```python
from build123d import *

# Parameters (mm, degrees)
BOSS_EXTRUDE1_DEPTH      = 47.625
BOSS_EXTRUDE1_DEPTH_BACK = 9.525
SKETCH2_R                = 9.525
CUT_EXTRUDE1_DEPTH       = 122.738617419


with BuildPart() as part:
    # Sketch1 → Boss-Extrude1 (new, two sides: drawn at the far end of the back side and taken through both)
    with BuildSketch(Plane.XY.offset(-BOSS_EXTRUDE1_DEPTH_BACK)):
        Polygon((-104.425717212, 293.558329543), (-143.022728413, 260.774121234), (-145.397980675, 262.922347723), (-106.481154517, 295.978206086), align=None)
    extrude(amount=BOSS_EXTRUDE1_DEPTH + BOSS_EXTRUDE1_DEPTH_BACK)

    # Sketch2 → Cut-Extrude1 (cut, through all)
    with BuildSketch(Plane(origin=(-188.610450601, 222.052019857, 0), x_dir=(0.762165840447724, 0.6473818283321017, 0), z_dir=(0.6473818283321017, -0.762165840447724, 0))):
        with Locations((85.054613578, 19.05)):
            Circle(SKETCH2_R)
        Polygon((110.454613578, -9.525), (88.229613578, -9.525), (88.229613578, -6.349999999), (91.404613578, -6.349999999), (91.404613578, -3.175), (97.754613578, -3.175), (97.754613578, 0), (110.454613578, 0), (113.679871945, 0), (113.679871945, -9.525), align=None)
        Polygon((59.813389382, -9.525), (82.038389382, -9.525), (82.038389382, -6.349999999), (78.863389382, -6.349999999), (78.863389382, -3.175), (72.513389382, -3.175), (72.513389382, 0), (59.813389382, 0), (54.830807426, 0), (54.830807426, -9.525), align=None)
        Polygon((110.454613578, 38.1), (118.192353476, 38.1), (118.192353476, 47.625), (110.454613578, 47.625), (88.229613578, 47.625), (88.229613578, 44.449999999), (91.404613578, 44.449999999), (91.404613578, 41.275), (97.754613578, 41.275), (97.754613578, 38.1), align=None)
        Polygon((59.393776038, 38.1), (50.339137781, 38.1), (50.339137781, 47.625), (59.393776038, 47.625), (81.618776038, 47.625), (81.618776038, 44.449999999), (78.443776038, 44.449999999), (78.443776038, 41.275), (72.093776038, 41.275), (72.093776038, 38.1), align=None)
    extrude(amount=-CUT_EXTRUDE1_DEPTH, mode=Mode.SUBTRACT)


solid = part.part
```
The listing builds one solid part. Answer for the finished solid, in the listing's coordinates (mm). A direction names the side the tool comes from. Round coordinates to 2 decimals unless told otherwise and drop trailing zeros. Loops run counter-clockwise (first coordinate to the right, second up) from the corner with the lowest first, then second, coordinate; pieces in that order, holes last.
1) For faces 1 (the face through (-127.1, 276.36, -7.96)), 2 (the face through (-118, 284, 41.275)), 3 (the face through (-118, 284, -3.175)), determine the directions among +Z, -Z, +X, -X, +Y, -Y from which every point of the face is accessible in a straight line to the end or side of a thin tool.
Outcome:
face 1: -Z, -X, -Y
face 2: +Z, +X, +Y
face 3: -Z, +X, +Y
2) Given P1, Ø7, axis at x = -116.5, y = 284.5, coming from the +Z side (3 decimals); P2, Ø7, axis at x = -119, y = 285, coming from the -Z side; P3, Ø8.5, axis at x = -108.5, y = 290.5, coming from the -Z side, each flat-ended and moving along its own axis, determine where each tip first touches the part or whether it passes through.
Outcome:
P1: stops at z = 41.275
P2: stops at z = -6.35
P3: stops at z = 0
3) A cutting plane is placed at D-D on y = 264.5. Determine the outline of the cut face in (x, z), plus the area to 3 significant figures.
Outcome:
outline: (-143.54, 0) - (-138.64, 0) - (-138.64, 38.1) - (-143.54, 38.1) - close
area: 187 mm2
4) Consider line 1 (Z direction, x = -133, y = 273) (3 decimals); line 2 (Y direction, x = -134, z = 33); line 3 (X direction, y = 286.5, z = 25). Determine where each line is inside the solid, lowest interval first.
Outcome:
line 1: z = -3.175 to 41.275
line 2: y = 268.44 to 272.6
line 3: x = -117.64 to -112.74
5) A cutting plane is placed at B-B on x = -115.5. Determine the outline of the cut face in (y, z) (3 decimals).
Outcome:
outline: (284.152, -3.175) - (286.979, -3.175) - (286.979, 0) - (288.318, 0) - (288.318, 38.1) - (286.979, 38.1) - (286.979, 41.275) - (284.152, 41.275) - close
6) A cutting plane is placed at A-A on z = 15.5. Determine the outline of the cut face in (x, y), plus the area to 3 significant figures.
Outcome:
outline: (-145.4, 262.92) - (-143.02, 260.77) - (-130.52, 271.39) - (-132.58, 273.81) - close; (-119.1, 285.26) - (-117.05, 282.84) - (-104.43, 293.56) - (-106.48, 295.98) - close
area: 105 mm2
7) A cutting plane is placed at C-C on z = 39. Determine the outline of the cut face in (x, y).
Outcome:
outline: (-135.72, 271.14) - (-133.66, 268.72) - (-114.11, 285.34) - (-116.16, 287.76) - close
